```python
from build123d import *

# Parameters (mm, degrees)
BOSS_EXTRUDE1_DEPTH = 4.8
SKETCH3_R           = 2.675
BOSS_EXTRUDE2_DEPTH = 28.7
FILLET1_R           = 0.25


with BuildPart() as part:
    # Sketch2 → Boss-Extrude1 (new body)
    with BuildSketch(Plane(origin=(0, 0, 0), x_dir=(1, 0, 0), z_dir=(0, 1, 0))):
        Polygon((-2.3375, 4.048668763), (-4.675, 0), (-2.3375, -4.048668763), (2.3375, -4.048668763), (4.675, 0), (2.3375, 4.048668763), align=None)
    extrude(amount=BOSS_EXTRUDE1_DEPTH)

    # Sketch3 → Boss-Extrude2 (add)
    with BuildSketch(Plane.XZ):
        with Locations(Location((0, 0, 0), (0, 0, 270))):
            Circle(SKETCH3_R)
    extrude(amount=BOSS_EXTRUDE2_DEPTH)

    # Fillet1
    fillet1_edges = [part.edges().sort_by_distance(p)[0] for p in [
        (0, 0, 2.675),
    ]]
    fillet(fillet1_edges, radius=FILLET1_R)


solid = part.part
```
CAD build for the part. Positions are in the model's coordinates, mm. A direction names the side the tool comes from. Coordinates: 2 decimals unless noted, no trailing zeros. Order: outer loops, then holes, each group sorted by start corner. A loop starts at its lowest first (then second) coordinate and runs counter-clockwise, first axis right, second up. Notation, with made-up numbers: M 56,12.5 L 62,12.5 A17 cw 62,40.5 Z; hole C 48.25,-22 d1. An arc over 180 degrees is marked long. Answer as CSV lines item,"result".
1) Flat gauge pins, fed straight in: P1, Ø1, axis at x = -2.5, y = -21.5, coming from the +Z side; P2, Ø4, axis at x = -2, y = -3.5, coming from the +Z side (3 decimals); P3, Ø1.5, axis at x = 1.5, y = -10.5, coming from the -Z side. Where does each tip first touch, or does it go through?
Verdict:
P1,"z = 1.78"
P2,"z = 2.675"
P3,"z = -2.57"
2) 3-axis set-ups, long thin cutter, end or side, ignore diameter. For faces 1 (the flat face through (-3.52, 2.37, 2)), 2 (the cylindrical face through (-2.61, -14.28, 0.58)): which of +Z, -Z, +X, -X, +Y, -Y reach the whole face in a straight line?
Verdict:
face 1,"+Z, -X, +Y, -Y"
face 2,"-Y"
3) Cut at A-A (x = 0). List the corners of the cut face in (y, z) (3 decimals), then the cut area to 3 significant figures.
Verdict:
outline,"M -28.7,-2.675 L -0.25,-2.675 A0.25 cw 0,-2.925 L 0,-4.049 L 4.8,-4.049 L 4.8,4.049 L 0,4.049 L 0,2.925 A0.25 cw -0.25,2.675 L -28.7,2.675 Z"
area,"192 mm2"
4) Cut at B-B (y = -7.5). List the corners of the cut face in (x, z) (3 decimals), then the cut area to 3 significant figures.
Verdict:
outline,"C 0,0 d5.35"
area,"22.5 mm2"
5) Drill centre lines: L1, parallel to Y at x = -2.25, z = 2.5; L2, parallel to Z at x = 0.25, y = -4.5; L3, parallel to Z at x = -1.25, y = -7.5. Where is each one in solid material? Low to high. Write a range as from..to.
Verdict:
L1,"0..4.8"
L2,"-2.66..2.66"
L3,"-2.36..2.36"
